```python
from build123d import *
from build123d.topology import SkipClean

# Parameters (mm, degrees)
SKETCH_1_R               = 2.4999999999999982
SKETCH_1_R_2             = 2.4999999999999947
SKETCH_1_R_3             = 2.5
EXTRUDE_1_DEPTH          = 5
EXTRUDE_START            = 12.8
SKETCH_2_R               = 5.000000000000004
SKETCH_2_R_2             = 2.4999999999999947
SKETCH_2_R_3             = 5
SKETCH_2_R_4             = 2.5
EXTRUDE_2_DEPTH          = 12.8
SKETCH_3_R               = 1.5000000000000007
CUT_EXTRUDE_1_DEPTH      = 13
EXTRUDE_START_2          = -5
EXTRUDE_3_DEPTH          = 5
FILLET_1_R               = 2
CUT_EXTRUDE_2_DEPTH      = 16
CUT_EXTRUDE_2_DEPTH_BACK = 10
CUT_EXTRUDE_START        = 14.000000000000002
SKETCH_7_R               = 5
CUT_EXTRUDE_3_DEPTH      = 14.000000000000002


with BuildPart() as part:
    # 草图1 → 凸台-拉伸1 (new body)
    with BuildSketch(Plane.XY):
        with BuildLine():
            Line((6.1e-16, -5), (-40, -5.000000000000006))
            ThreePointArc((-40, -5.000000000000006), (-45, -4.29e-15), (-40, 4.999999999999996))
            Line((-40, 4.999999999999996), (-6.1e-16, 5))
            ThreePointArc((-6.1e-16, 5), (5, 0), (6.1e-16, -5))
        make_face()
        with Locations((-20, -2.45e-15)):
            Circle(SKETCH_1_R, mode=Mode.SUBTRACT)
        with Locations((-40, -4.9e-15)):
            Circle(SKETCH_1_R_2, mode=Mode.SUBTRACT)
        Circle(SKETCH_1_R_3, mode=Mode.SUBTRACT)
    extrude(amount=EXTRUDE_1_DEPTH)

    # 草图2 → 凸台-拉伸2 (add)
    # profile 1 of 2: a face of its own
    with SkipClean():  # the faces are left unmerged after this step: merging them gives an invalid solid
        with BuildSketch(Plane(origin=(0, 0, 0), x_dir=(-1, 0, 0), z_dir=(0, 0, -1)).offset(EXTRUDE_START)):
            with Locations((40, -4.9e-15)):
                Circle(SKETCH_2_R)
            with Locations((40, -4.9e-15)):
                Circle(SKETCH_2_R_2, mode=Mode.SUBTRACT)
        # profile 2 of 2: a face of its own
        with BuildSketch(Plane(origin=(0, 0, 0), x_dir=(-1, 0, 0), z_dir=(0, 0, -1)).offset(EXTRUDE_START)):
            Circle(SKETCH_2_R_3)
            Circle(SKETCH_2_R_4, mode=Mode.SUBTRACT)
        extrude(amount=-EXTRUDE_2_DEPTH)

    # 草图3 → 切除-拉伸1 (cut)
    with SkipClean():  # the faces are left unmerged after this step: merging them gives an invalid solid
        with BuildSketch(Plane.XY.offset(5)):
            with Locations((-26.000000000000004, -2.45e-15)):
                Circle(SKETCH_3_R)
            with Locations((-13.999999999999998, -2.4e-16)):
                Circle(SKETCH_3_R)
        extrude(amount=-CUT_EXTRUDE_1_DEPTH, mode=Mode.SUBTRACT)

    # 草图4 → 凸台-拉伸3 (add)
    with SkipClean():  # the faces are left unmerged after this step: merging them gives an invalid solid
        with BuildSketch(Plane.XY.offset(5).offset(EXTRUDE_START_2)):
            with BuildLine():
                Line((-29.484888992731253, 3.168103659220378), (-10.515111007268752, 3.168103659220378))
                ThreePointArc((-10.515111007268752, 3.168103659220378), (-20, 9.999999999999996), (-29.484888992731253, 3.168103659220378))
            make_face()
            with BuildLine():
                Line((-29.548830353481478, -2.969821354969149), (-10.451169646518524, -2.969821354969149))
                ThreePointArc((-10.451169646518524, -2.969821354969149), (-20, -10), (-29.548830353481478, -2.969821354969149))
            make_face()
        extrude(amount=EXTRUDE_3_DEPTH)

    # 圆角1
    fillet_1_edges = [part.edges().sort_by_distance(p)[0] for p in [
        (-11.339745962155616, -5.000000000000002, 2.5),
        (-28.660254037844382, -5.000000000000005, 2.5),
        (-28.660254037844386, 4.999999999999997, 2.5),
        (-11.339745962155614, 4.999999999999999, 2.5),
    ]]
    fillet(fillet_1_edges, radius=FILLET_1_R)

    # 草图6 → 切除-拉伸2 (cut, two sides: drawn at the far end of the back side and taken through both)
    with SkipClean():  # the faces are left unmerged after this step: merging them gives an invalid solid
        with BuildSketch(Plane(origin=(0, 0, 0), x_dir=(-1, 0, 0), z_dir=(0, 0, -1)).offset(-CUT_EXTRUDE_2_DEPTH_BACK)):
            with BuildLine():
                Line((28.122328620674136, 5.83333333333333), (47.018648457175516, 5.83333333333333))
                Line((47.018648457175516, 5.83333333333333), (47.018648457175516, -5.833333333333338))
                Line((47.018648457175516, -5.833333333333338), (28.122328620674132, -5.833333333333338))
                ThreePointArc((28.122328620674132, -5.833333333333338), (30, -4.67e-15), (28.122328620674136, 5.83333333333333))
            make_face()
        extrude(amount=CUT_EXTRUDE_2_DEPTH + CUT_EXTRUDE_2_DEPTH_BACK, mode=Mode.SUBTRACT)

    # 草图7 → 切除-拉伸3 (cut)
    with SkipClean():  # the faces are left unmerged after this step: merging them gives an invalid solid
        with BuildSketch(Plane(origin=(0, 0, 0), x_dir=(-1, 0, 0), z_dir=(0, 0, -1)).offset(CUT_EXTRUDE_START)):
            Circle(SKETCH_7_R)
        extrude(amount=-CUT_EXTRUDE_3_DEPTH, mode=Mode.SUBTRACT)


solid = part.part
```
Could you check a few things on this model? Use its own coordinates, in mm. A direction names the side the tool comes from. Coordinates: 2 decimals unless noted, no trailing zeros. Loops run counter-clockwise (first coordinate to the right, second up) from the corner with the lowest first, then second, coordinate; pieces in that order, holes last. Notation, with made-up numbers: M 38.25,-17 L 68.25,-17 A26 cw 68.25,1 Z; hole C -16.75,68 d4. An arc over 180 degrees is marked long. Put each result on its own line as item: value. Start each with the question number.
(1) Suppose I cut it at A-A on y = 0. Please give me the cut outline in (x, z), then the cut area to 3 significant figures.
(2) Suppose I cut it at D-D on x = -20. Please give me the cut outline in (y, z).
(3) I need wall thicknesses on line 1 (X direction, y = -2.25, z = 4.1); line 2 (Y direction, x = -21, z = 1.4); line 3 (Y direction, x = -5, z = 4.85). Which ranges of each line are inside material? Lowest first, please. Write a range as from..to.
(4) Suppose I cut it at B-B on x = -26. Please give me the cut outline in (y, z).
(5) For faces 4 (the face through (-5, -5, 2)), 5 (the face through (-15.5, 0.07, 2.54)), 6 (the face through (-5, 5, 2)), which set-ups out of +Z, -Z, +X, -X, +Y, -Y let a thin tool reach every point of the face, with its end or its side?
(6) Suppose I cut it at C-C on z = 1. Please give me the cut outline in (x, y), then the cut area to 3 significant figures.
(7) Thinking about a two-plate mould opening in Y: for faces 1 (the face through (-22.5, 0.1, 2.5)), 2 (the face through (5, 0, 2)), 3 (the face through (-17, 0, 5)), which applies, pulls with the +Y half, pulls with the -Y half, needs draft (parallel to the pull), parting line crosses it, or undercut?
(8) Will these pins go through, and if not, where does the flat tip stop? P1, Ø1, axis at y = -6, z = 3, coming from the -X side; P2, Ø1.8, axis at x = -26, y = 0, coming from the +Z side; P3, Ø2.5, axis at x = -6, z = 3, coming from the -Y side.
Solutions:
1. outline: M -30,0 L -27.5,0 L -27.5,5 L -30,5 Z; M -24.5,0 L -22.5,0 L -22.5,5 L -24.5,5 Z; M -17.5,0 L -15.5,0 L -15.5,5 L -17.5,5 Z; M -12.5,0 L -2.5,0 L -2.5,5 L -12.5,5 Z; M 2.5,0 L 5,0 L 5,5 L 2.5,5 Z
1. area: 95.0 mm2
2. outline: M -10,0 L -2.5,0 L -2.5,5 L -10,5 Z; M 2.5,0 L 10,0 L 10,5 L 2.5,5 Z
3. line 1: x = -29.74..-21.09, -18.91..-1.09, 1.09..4.47
3. line 2: y = -9.95..-2.29, 2.29..9.95
3. line 3: y = -5..5
4. outline: M -8,0 L -1.5,0 L -1.5,5 L -8,5 Z; M 1.5,0 L 8,0 L 8,5 L 1.5,5 Z
5. face 4: +Z, -Z, +X, -Y
5. face 5: +Z, -Z
5. face 6: +Z, -Z, +X, +Y
6. outline: M -11.88,-5.83 A2 cw -10.25,-5 L 0,-5 A5 ccw 0,5 L -10.25,5 A2 cw -11.88,5.83 A10 ccw long Z; hole C -26,0 d3; hole C -20,0 d5; hole C -14,0 d3; hole C 0,0 d5
6. area: 405 mm2
7. face 1: undercut
7. face 2: parting line crosses it
7. face 3: needs draft
8. P1: stops at x = -28.35
8. P2: passes through
8. P3: stops at y = -5
